Check sheet for the drawn part. Datum: minimum x, y, z corner. Units: mm. A direction names the side the tool comes from. Coordinates: 2 decimals unless noted, no trailing zeros. Order: outer loops, then holes, each group sorted by start corner. A loop starts at its lowest first (then second) coordinate and runs counter-clockwise, first axis right, second up. Notation, with made-up numbers: (-23.5, 31.25) - (8.5, 31.25) arc R21 cw to (8.5, 61.25) - close; hole circle Ø11 at (70, 47.25). An arc over 180 degrees is marked (long way). Answer as CSV lines item,"result". Start each with the question number.
1. Mould release check, pull along Y, two halves, no side actions. Record for the marked faces 5, 6, 7 and 8: pulls with the +Y half, pulls with the -Y half, needs draft (parallel to the pull), parting line crosses it, or undercut.
2. Section check D-D (y = 61.5). Record the cut outline in (x, z).
3. Section check A-A (z = 27.5). Record the cut outline in (x, y), and give its area (3 significant figures).
4. Go/stop test with flat-tipped pins: pin 1 (13.5 mm diameter, centred on x = 60, y = 10, fed in from +Z); pin 2 (5 mm diameter, centred on y = 66, z = 7, fed in from -X); pin 3 (6 mm diameter, centred on x = 58.5, y = 9.5, fed in from -Z). Record where each tip stops, or that it passes through.
5. Material ranges on L1, parallel to Y at x = 60, z = 21.5; L2, parallel to X at y = 62, z = 20, recorded low to high. Write a range as [from, to].
6. Section check C-C (x = 4). Record the cut outline in (y, z).
7. Set-up check for the marked faces 1, 2, 3 and 4: record each of +Z, -Z, +X, -X, +Y, -Y from which the full face is reachable in a straight line by a thin tool's end or side.
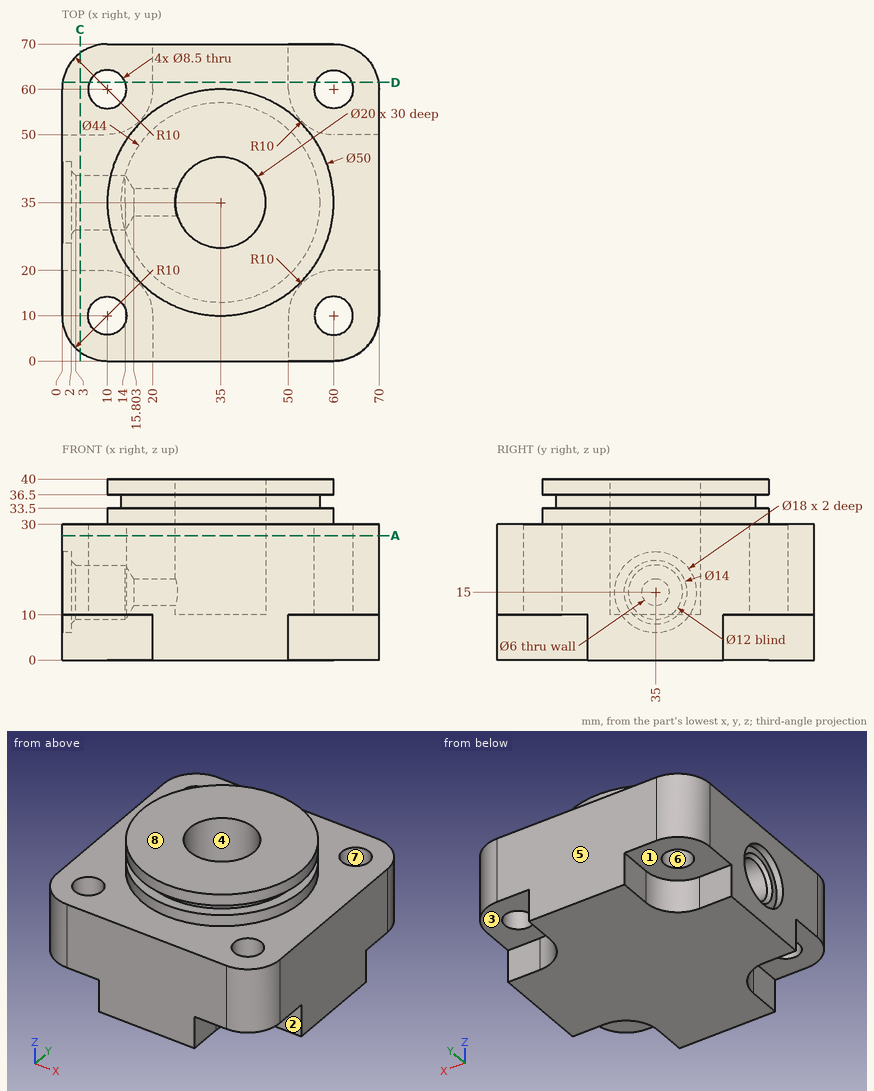
Evaluation:
1,face 5,"pulls with the +Y half"
1,face 6,"undercut"
1,face 7,"undercut"
1,face 8,"needs draft"
2,outline,"(0.11, 10) - (6.02, 10) - (6.02, 30) - (0.11, 30) - close; (13.98, 10) - (20, 10) - (20, 0) - (50, 0) - (50, 10) - (56.02, 10) - (56.02, 30) - (13.98, 30) - close; (63.98, 10) - (69.89, 10) - (69.89, 30) - (63.98, 30) - close"
3,outline,"(0, 10) arc R10 ccw to (10, 0) - (60, 0) arc R10 ccw to (70, 10) - (70, 60) arc R10 ccw to (60, 70) - (10, 70) arc R10 ccw to (0, 60) - close; hole circle Ø8.5 at (10, 10); hole circle Ø8.5 at (10, 60); hole circle Ø20 at (35, 35); hole circle Ø8.5 at (60, 10); hole circle Ø8.5 at (60, 60)"
3,area,"4,270 mm²"
4,pin 1,"stops at z = 30"
4,pin 2,"stops at x = 20"
4,pin 3,"stops at z = 10"
5,L1,"y = [0, 5.75], [14.25, 55.75], [64.25, 70]"
5,L2,"x = [0.2, 6.25], [13.75, 56.25], [63.75, 69.8]"
6,outline,"(2, 10) - (20, 10) - (20, 0) - (50, 0) - (50, 10) - (68, 10) - (68, 30) - (2, 30) - close; hole circle Ø12 at (35, 15)"
7,face 1,"-Z, -X, +Y"
7,face 2,"-Z, +X, -Y"
7,face 3,"-Z, +X, +Y"
7,face 4,"+Z"
